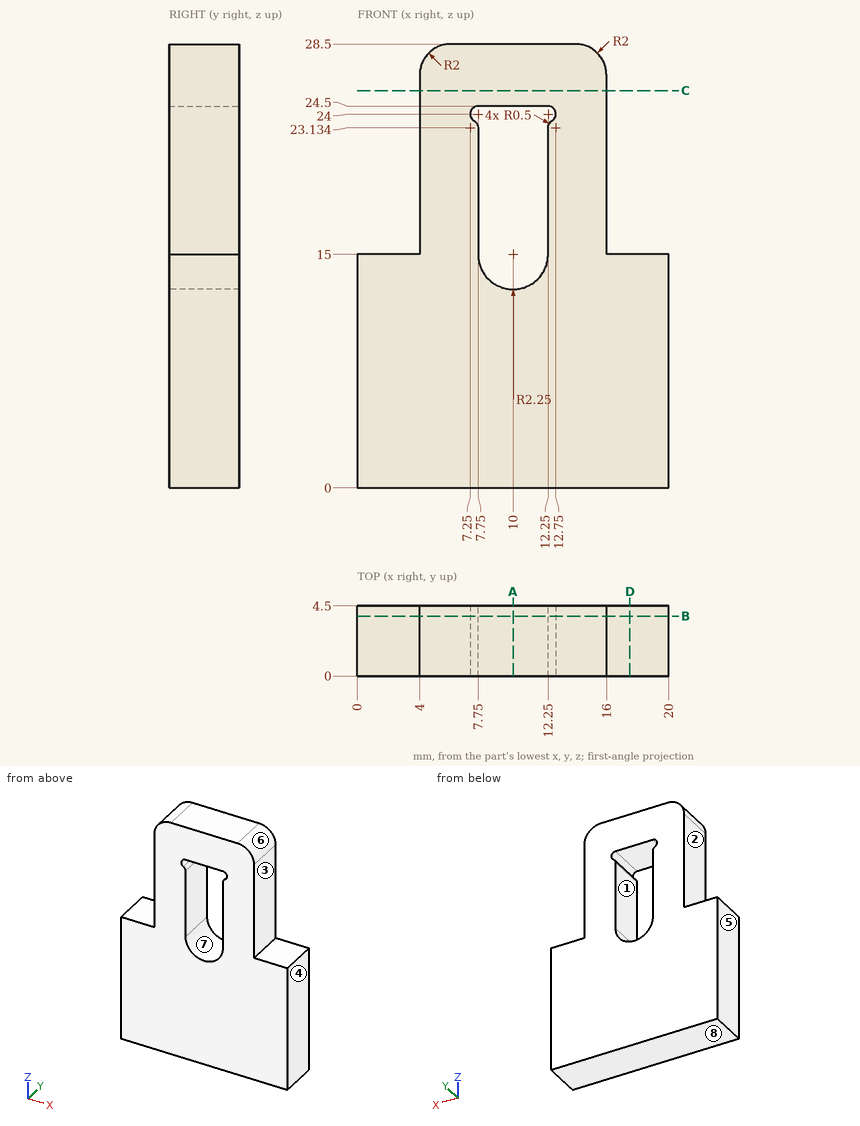
Input: dimensioned drawing with shaded views. Units: mm. Origin: part minimum x, y, z. A direction names the side the tool comes from. Give positions to 0.01 mm unless a question says otherwise; leave off trailing zeros. Write each loop counter-clockwise with the first axis right and the second up, starting at its lowest first coordinate (ties: lowest second). Pieces come first, ordered by that corner, then holes.
Q1. Section A-A, the plane x = 10. Output: boundary loops of the cut face in (y, z).
Q2. Section C-C, the plane z = 25.5. Output: boundary loops of the cut face in (x, y).
Q3. Section D-D, the plane x = 17.5. Output: boundary loops of the cut face in (y, z), plus the area to 3 significant figures.
Q4. First-contact query: P1, Ø1.2, axis at x = 2.5, y = 1.5, coming from the +Z side; P2, Ø1.5, axis at y = 3, z = 21.5, coming from the +X side. Flat tips, straight axial feed; report the tip coordinate or a pass-through.
Q5. Set-up query: the marked faces 1, 2, 3, 4 and 5. Return all of +Z, -Z, +X, -X, +Y, -Y with unobstructed straight access to the full face (end or side cutting, diameter ignored); none if empty.
Q6. Pull-direction query (X, two-part tool) for the marked faces 6, 7 and 8; classes: pulls with the +X half, pulls with the -X half, needs draft (parallel to the pull), parting line crosses it, or undercut.
Q7. Section B-B, the plane y = 3.85. Output: boundary loops of the cut face in (x, z), plus the area to 3 significant figures.
Q8. Material intervals for probe 1 along X at (y, z) = (2.75, 21.25); probe 2 along Z at (x, y) = (18, 3.5); probe 3 along X at (y, z) = (2.45, 25.5), sorted ascending.
Filled in:
1. outline: (0, 0) - (4.5, 0) - (4.5, 12.75) - (0, 12.75) - close; (0, 24.5) - (4.5, 24.5) - (4.5, 28.5) - (0, 28.5) - close
2. outline: (4, 0) - (16, 0) - (16, 4.5) - (4, 4.5) - close
3. outline: (0, 0) - (4.5, 0) - (4.5, 15) - (0, 15) - close
3. area: 67.5 mm2
4. P1: stops at z = 15
4. P2: stops at x = 16
5. face 1: +Y, -Y
5. face 2: +Z, -X, +Y, -Y
5. face 3: +Z, +X, +Y, -Y
5. face 4: +Z, -Z, +X, +Y, -Y
5. face 5: +Z, -Z, -X, +Y, -Y
6. face 6: pulls with the +X half
6. face 7: undercut
6. face 8: needs draft
7. outline: (0, 0) - (20, 0) - (20, 15) - (16, 15) - (16, 26.5) arc R2 ccw to (14, 28.5) - (6, 28.5) arc R2 ccw to (4, 26.5) - (4, 15) - (0, 15) - close; hole (7.5, 23.57) arc R0.5 cw to (7.75, 23.13) - (7.75, 15) arc R2.25 ccw to (12.25, 15) - (12.25, 23.13) arc R0.5 cw to (12.5, 23.57) arc R0.5 ccw to (12.25, 24.5) - (7.75, 24.5) arc R0.5 ccw to start
7. area: 409 mm2
8. probe 1: x = 4 to 7.75, 12.25 to 16
8. probe 2: z = 0 to 15
8. probe 3: x = 4 to 16
